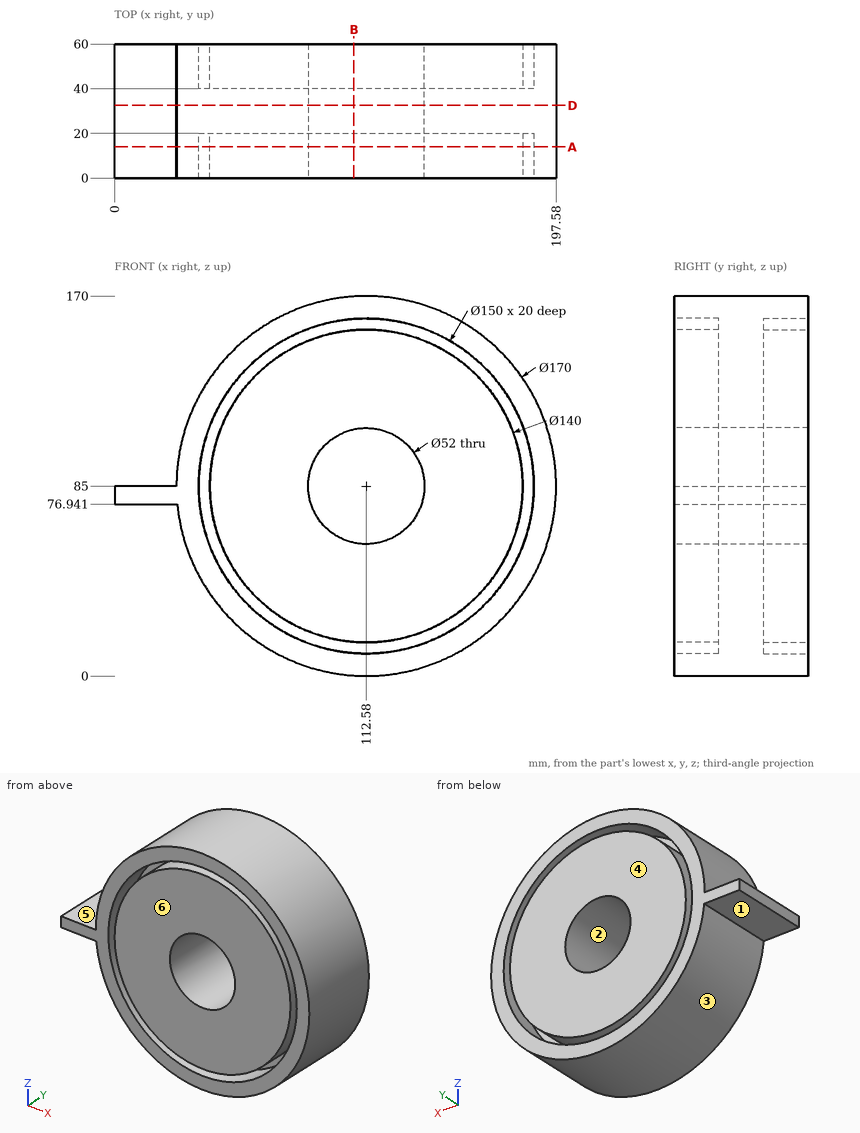
For this review, use the dimensioned drawing (mm, ordinates from the lowest corner) and the shaded views. A direction names the side the tool comes from. Round coordinates to 2 decimals unless told otherwise and drop trailing zeros. Write each loop counter-clockwise with the first axis right and the second up, starting at its lowest first coordinate (ties: lowest second). Pieces come first, ordered by that corner, then holes. Notation, with made-up numbers: (38.5, -18.5) - (42.5, -18.5) arc R23 ccw to (42.5, 3.5) - close; hole circle Ø9 at (-38.75, 40.25). An arc over 180 degrees is marked (long way). Answer as CSV lines item,"result". Start each with the question number.
(1) We need section D-D on y = 32.5. State the section outline as (x, z) points.
(2) For the marked faces 5 and 6, list the 3-axis set-ups (+Z, -Z, +X, -X, +Y, -Y) from which the entire face can be reached by the end or side of a thin tool; tool diameter is ignored.
(3) For pin 1 Ø12 at (x, z) = (99, 42.5) entering from -Y; pin 2 Ø10 at (x, y) = (35.5, 12) entering from -Z; pin 3 Ø3 at (x, y) = (141.5, 26) entering from +Z; pin 4 Ø10 at (x, y) = (81.5, 18) entering from +Z, all flat-tipped, find the tip position at first contact; note any pin that passes through.
(4) We need section A-A on y = 14. State the section outline as (x, z) points.
(5) We need section B-B on x = 107. State the section outline as (y, z) points.
(6) Draft analysis for pull direction Z (two halves, no side actions). For the marked faces 1, 2, 3 and 4, state which applies: pulls with the +Z half, pulls with the -Z half, needs draft (parallel to the pull), parting line crosses it, or undercut.
(7) To check wall thickness, follow line 1 (X direction, y = 56, z = 53); line 2 (X direction, y = 12, z = 141) (1 decimal); line 3 (Z direction, x = 167.5, y = 15) (1 decimal). State the ranges of each line that lie inside material, in increasing order.
Worked answers:
1,outline,"(0, 76.94) - (27.96, 76.94) arc R85 ccw (long way) to (27.58, 85) - (0, 85) - close; hole circle Ø52 at (112.58, 85)"
2,face 5,"+Z, -X, +Y, -Y"
2,face 6,"+Z, -Z, +X, -X, -Y"
3,pin 1,"y = 0"
3,pin 2,"z = 39.95"
3,pin 3,"z = 165.46"
3,pin 4,"z = 165.9"
4,outline,"(0, 76.94) - (27.96, 76.94) arc R85 ccw (long way) to (27.58, 85) - (0, 85) - close; circle Ø140 at (112.58, 85); hole circle Ø150 at (112.58, 85); hole circle Ø52 at (112.58, 85)"
5,outline,"(0, 0.18) - (60, 0.18) - (60, 10.21) - (40, 10.21) - (40, 15.22) - (60, 15.22) - (60, 59.61) - (0, 59.61) - (0, 15.22) - (20, 15.22) - (20, 10.21) - (0, 10.21) - close; (0, 110.39) - (60, 110.39) - (60, 154.78) - (40, 154.78) - (40, 159.79) - (60, 159.79) - (60, 169.82) - (0, 169.82) - (0, 159.79) - (20, 159.79) - (20, 154.78) - (0, 154.78) - close"
6,face 1,"pulls with the -Z half"
6,face 2,"undercut"
6,face 3,"parting line crosses it"
6,face 4,"needs draft"
7,line 1,"33.83 to 44.75, 50.32 to 174.84, 180.41 to 191.33"
7,line 2,"48.6 to 62.7, 70.6 to 154.6, 162.5 to 176.5"
7,line 3,"20.1 to 33.9, 41.6 to 128.4, 136.1 to 149.9"
